```python
from build123d import *

# Parameters (mm, degrees)
SKETCH024_W     = 95
SKETCH024_H     = 95
PAD016_DEPTH    = 5
PAD017_DEPTH    = 95
SKETCH029_R     = 30
POCKET009_DEPTH = 104.501
FILLET022_R     = 5
FILLET023_R     = 2


with BuildPart() as part:
    # Sketch024 → Pad016 (new body)
    with BuildSketch(Plane.XY):
        Rectangle(SKETCH024_W, SKETCH024_H)
    extrude(amount=PAD016_DEPTH)

    # Sketch025 (on DatumPlane) → Pad017 (join)
    with BuildSketch(Plane(origin=(0, 47.5, 0), x_dir=(-1, 0, 0), z_dir=(0, 1, 0))):
        Polygon((-47, 5), (-17, 56.961524), (-14, 56.961524), (-44, 5), align=None)
        Polygon((-22, 5), (8, 56.961524), (11, 56.961524), (-19, 5), align=None)
        Polygon((1, 5), (31, 56.961524), (34, 56.961524), (4, 5), align=None)
        Polygon((24, 5), (54, 56.961524), (57, 56.961524), (27, 5), align=None)
    extrude(amount=-PAD017_DEPTH)

    # Sketch029 (on DatumPlane) → Pocket009 (cut, through all)
    with BuildSketch(Plane.YZ.offset(47.5)):
        with Locations((0, 60)):
            Circle(SKETCH029_R)
    extrude(amount=-POCKET009_DEPTH, mode=Mode.SUBTRACT)

    # Fillet022
    fillet022_edges = [part.edges().sort_by_distance(p)[0] for p in [
        (15.5, -47.5, 56.961524),
        (15.5, -29.845731, 56.961524),
        (-9.5, -47.5, 56.961524),
        (-9.5, -29.845731, 56.961524),
        (-32.5, -47.5, 56.961524),
        (-32.5, -29.845731, 56.961524),
        (-55.5, -47.5, 56.961524),
        (-55.5, -29.845731, 56.961524),
        (15.5, 29.845731, 56.961524),
        (15.5, 47.5, 56.961524),
        (-9.5, 29.845731, 56.961524),
        (-9.5, 47.5, 56.961524),
        (-32.5, 29.845731, 56.961524),
        (-32.5, 47.5, 56.961524),
        (-55.5, 29.845731, 56.961524),
        (-55.5, 47.5, 56.961524),
    ]]
    fillet(fillet022_edges, radius=FILLET022_R)

    # Fillet023
    fillet023_edges = [part.edges().sort_by_distance(p)[0] for p in [
        (0, -47.5, 0),
        (47.5, 0, 0),
        (0, 47.5, 0),
        (-47.5, 0, 0),
    ]]
    fillet(fillet023_edges, radius=FILLET023_R)


with BuildPart() as part_1:
    # Body011 placement: moved
    add(part.part.moved(Location((48, 233, 0))))


solid = part_1.part
```
Geometry check sheet. Reference: the model listing, model coordinates, mm. A direction names the side the tool comes from. Coordinates: 2 decimals unless noted, no trailing zeros. Order: outer loops, then holes, each group sorted by start corner. A loop starts at its lowest first (then second) coordinate and runs counter-clockwise, first axis right, second up. Notation, with made-up numbers: M 65,11.25 L 105,11.25 A16 cw 105,31.25 Z; hole C 24,-38 d4. An arc over 180 degrees is marked long. One line per question, with ' | ' between items. Start each with the question number.
Item 1: Cross-section at B-B on x = 72. Enter the section's corners in (y, z).
Item 2: Cross-section at C-C on y = 232. Enter the section's corners in (x, z).
Item 3: Material ranges on L1, parallel to X at y = 271.5, z = 6.5; L2, parallel to X at y = 263.5, z = 25; L3, parallel to Z at x = 52, y = 260, recorded low to high. Write a range as [from, to].
Item 4: Cross-section at A-A on z = 49.5. State how many separate pieces and enclosed holes the cut face has, then the cut area to 3 significant figures.
Item 5: Cross-section at D-D on z = 22. Enter the section's corners in (x, y).
Item 6: Gauge pin test, flat ends, axial feed: pin 1 (6 mm diameter, centred on y = 209.5, z = 13, fed in from -X); pin 2 (3 mm diameter, centred on x = 42, y = 223.5, fed in from +Z); pin 3 (4 mm diameter, centred on y = 241.5, z = 18, fed in from +X); pin 4 (8 mm diameter, centred on x = 58, z = 26, fed in from -Y). Record the tip position at first contact, or that the pin passes through.
Item 7: Set-up check for faces 1 (the cylindrical face through (-6.93, 202, 55.91)), 2 (the cylindrical face through (64.25, 186.93, 55.46)), 3 (the flat face through (9.123, 233.665, 25.571)), 4 (the flat face through (95.5, 232, 3)), 5 (the flat face through (35.543, 233.665, 24.844)): record each of +Z, -Z, +X, -X, +Y, -Y from which the full face is reachable in a straight line by a thin tool's end or side.
Item 8: Draft check along Y on faces 6 (the cylindrical face through (29.961, 229.843, 30.167)), 7 (the flat face through (16, 195, 56.962)), 8 (the cylindrical face through (-6.75, 279.07, 55.46)), 9 (the cylindrical face through (52.961, 229.843, 30.167)). Enter one of: pulls with the +Y half, pulls with the -Y half, needs draft (parallel to the pull), parting line crosses it, or undercut.
Findings:
1) outline: M 185.5,2 A2 ccw 187.5,0 L 278.5,0 A2 ccw 280.5,2 L 280.5,5 L 185.5,5 Z; M 185.5,39.64 L 210.97,39.64 A30 cw 207.11,44.84 L 185.5,44.84 Z; M 255.03,39.64 L 280.5,39.64 L 280.5,44.84 L 258.89,44.84 A30 cw Z
2) outline: M 0.5,2 A2 ccw 2.5,0 L 93.5,0 A2 ccw 95.5,2 L 95.5,5 L 95,5 L 80.56,30.02 L 77.56,30.02 L 92,5 L 70,5 L 55.56,30.02 L 52.56,30.02 L 67,5 L 47,5 L 32.56,30.02 L 29.56,30.02 L 44,5 L 24,5 L 9.56,30.02 L 6.56,30.02 L 21,5 L 0.5,5 Z
3) L1: x = [20.13, 23.13], [43.13, 46.13], [66.13, 69.13], [91.13, 94.13] | L2: x = [9.45, 12.45], [32.45, 35.45], [55.45, 58.45], [80.45, 83.45] | L3: z = [0, 5], [30.98, 36.18]
4) separate pieces: 8 | enclosed holes: 0 | area: 466 mm²
5) outline: M 11.19,185.5 L 14.19,185.5 L 14.19,280.5 L 11.19,280.5 Z; M 34.19,185.5 L 37.19,185.5 L 37.19,280.5 L 34.19,280.5 Z; M 57.19,185.5 L 60.19,185.5 L 60.19,280.5 L 57.19,280.5 Z; M 82.19,185.5 L 85.19,185.5 L 85.19,280.5 L 82.19,280.5 Z
6) pin 1: stops at x = 14.65 | pin 2: stops at z = 16.26 | pin 3: stops at x = 88.65 | pin 4: stops at y = 185.5
7) face 1: +Z, +X, -X | face 2: +Z, +X, -X, -Y | face 3: -X, +Y, -Y | face 4: +Z, -Z, +X, +Y, -Y | face 5: +Y, -Y
8) face 6: undercut | face 7: needs draft | face 8: pulls with the +Y half | face 9: undercut
